from build123d import *

# Parameters (mm, degrees)
SKETCH1_R             = 4
SKETCH1_R_2           = 2
BOSS_EXTRUDE1_DEPTH   = 2
BOSS_EXTRUDE1_2_DEPTH = 2
SKETCH2_W             = 60
SKETCH2_H             = 16
SKETCH2_R             = 2.25
BOSS_EXTRUDE2_DEPTH   = 3
SKETCH3_R             = 1.6
CUT_EXTRUDE1_DEPTH    = 10


with BuildPart() as part:
    # Sketch1 → Boss-Extrude1 (new body)
    with BuildSketch(Plane(origin=(0, 0, 0), x_dir=(1, 0, 0), z_dir=(0, 1, 0))):
        Circle(SKETCH1_R)
        Circle(SKETCH1_R_2, mode=Mode.SUBTRACT)
    extrude(amount=BOSS_EXTRUDE1_DEPTH)



with BuildPart() as body_2:
    # Sketch1 → Boss-Extrude1 2 (new body)
    with BuildSketch(Plane(origin=(0, 0, 0), x_dir=(1, 0, 0), z_dir=(0, 1, 0))):
        with Locations((19, 0)):
            Circle(SKETCH1_R)
        with Locations((19, 0)):
            Circle(SKETCH1_R_2, mode=Mode.SUBTRACT)
    extrude(amount=BOSS_EXTRUDE1_2_DEPTH)


with BuildPart() as part_1:
    add(part.part)

    add(body_2.part)  # Boss-Extrude2 merges body 2
    # Sketch2 → Boss-Extrude2 (add)
    with BuildSketch(Plane.XZ):
        with Locations((12, -4)):
            Rectangle(SKETCH2_W, SKETCH2_H)
        with Locations((-8, -4)):
            Circle(SKETCH2_R, mode=Mode.SUBTRACT)
        with Locations((32, -4)):
            Circle(SKETCH2_R, mode=Mode.SUBTRACT)
    extrude(amount=BOSS_EXTRUDE2_DEPTH)

    # Sketch3 → Cut-Extrude1 (cut)
    with BuildSketch(Plane(origin=(0, 2, 0), x_dir=(1, 0, 0), z_dir=(0, 1, 0))):
        Circle(SKETCH3_R)
        with Locations((19, 0)):
            Circle(SKETCH3_R)
    extrude(amount=-CUT_EXTRUDE1_DEPTH, mode=Mode.SUBTRACT)


solid = part_1.part
Verification items for the finished model (mm, model axes). A direction names the side the tool comes from. Give positions to 0.01 mm unless a question says otherwise; leave off trailing zeros. Loops run counter-clockwise (first coordinate to the right, second up) from the corner with the lowest first, then second, coordinate; pieces in that order, holes last.
1) Sectioned sample at C-C, the plane z = 0. Enter the section's corners in (x, y), then the cut area to 3 significant figures.
2) Sectioned sample at B-B, the plane y = -1.85. Enter the section's corners in (x, z).
3) Sectioned sample at D-D, the plane z = -10.75. Enter the section's corners in (x, y).
4) Draft check along Z on faces 1 (the cylindrical face through (-0.867, 0.986, 3.905)), 2 (the cylindrical face through (-9.786, -1.479, -5.369)), 3 (the flat face through (-2, 2, 1)). Enter one of: pulls with the +Z half, pulls with the -Z half, needs draft (parallel to the pull), parting line crosses it, or undercut.
5) Depth check by flat-ended pin: pin 1 Ø1.2 at (x, z) = (19.5, -0.5) entering from +Y; pin 2 Ø2 at (x, z) = (28.5, 0) entering from +Y. Enter the tip coordinate at first touch or a pass-through.
6) Sectioned sample at A-A, the plane x = -8. Enter the section's corners in (y, z).
7) Set-up check for faces 4 (the cylindrical face through (17.4, 1, 1.2)), 5 (the flat face through (12, -1, 4)): record each of +Z, -Z, +X, -X, +Y, -Y from which the full face is reachable in a straight line by a thin tool's end or side.
8) Thickness scan on line 1 along X through (y, z) = (-1.2, 1); line 2 along X through (y, z) = (1.45, 1.5); line 3 along Z through (x, y) = (19, -1.1). Record the ranges inside material, lowest first.
Answers:
1. outline: (-18, -3) - (-1.6, -3) - (-1.6, 0) - (-2, 0) - (-2, 2) - (-4, 2) - (-4, 0) - (-18, 0) - close; (1.6, -3) - (17.4, -3) - (17.4, 0) - (17, 0) - (17, 2) - (15, 2) - (15, 0) - (4, 0) - (4, 2) - (2, 2) - (2, 0) - (1.6, 0) - close; (20.6, -3) - (42, -3) - (42, 0) - (23, 0) - (23, 2) - (21, 2) - (21, 0) - (20.6, 0) - close
1. area: 177 mm2
2. outline: (-18, -12) - (42, -12) - (42, 4) - (-18, 4) - close; hole circle Ø4.5 at (-8, -4); hole circle Ø3.2 at (0, 0); hole circle Ø3.2 at (19, 0); hole circle Ø4.5 at (32, -4)
3. outline: (-18, -3) - (42, -3) - (42, 0) - (-18, 0) - close
4. face 1: parting line crosses it
4. face 2: undercut
4. face 3: needs draft
5. pin 1: passes through
5. pin 2: stops at y = 0
6. outline: (-3, -12) - (0, -12) - (0, -6.25) - (-3, -6.25) - close; (-3, -1.75) - (0, -1.75) - (0, 4) - (-3, 4) - close
7. face 4: +Y
7. face 5: +Z, +X, -X, +Y, -Y
8. line 1: x = -18 to -1.25, 1.25 to 17.75, 20.25 to 42
8. line 2: x = -3.71 to -1.32, 1.32 to 3.71, 15.29 to 17.68, 20.32 to 22.71
8. line 3: z = -12 to -1.6, 1.6 to 4
